Verification items for the finished model (mm, model axes). Face numbers are marked on the shaded views. A direction names the side the tool comes from. Coordinates: 2 decimals unless noted, no trailing zeros. Loops run counter-clockwise (first coordinate to the right, second up) from the corner with the lowest first, then second, coordinate; pieces in that order, holes last. Notation, with made-up numbers: (60.25, 1.5) - (105.25, 1.5) arc R15 ccw to (105.25, 8.5) - close; hole circle Ø6 at (-29, 11.5). An arc over 180 degrees is marked (long way). One line per item, written item: value. Start each with the question number.
(1) Section check C-C (x = 424.5). Record the boundary of the cut face in (y, z), plus the area to 3 significant figures.
(2) Gauge pin test, flat end, axial feed: P1, Ø8, axis at y = 115.5, z = 32, coming from the -X side. Record the tip position at first contact, or that the pin passes through.
(3) Draft check along Y on the marked faces 3, 4, 5 and 6. Enter one of: +Y half, -Y half, draft (parallel to the pull), parting line (faces both ways), or undercut.
(4) Section check A-A (z = 51). Record the boundary of the cut face in (x, y).
(5) Set-up check for the marked faces 1 and 2: record each of +Z, -Z, +X, -X, +Y, -Y from which the full face is reachable in a straight line by a thin tool's end or side.
(6) Thickness scan on probe 1 along Y at (x, z) = (173, 24); probe 2 along X at (y, z) = (34.5, 9); probe 3 along Y at (x, z) = (623, 72.5). Record the ranges inside material, lowest first. Write a range as [from, to].
(7) Section check B-B (y = -10.5). Record the boundary of the cut face in (x, z), plus the area to 3 significant figures.
Autodesk Inventor part; units mm, degrees
ref_plane "YZ Plane" through (0, 0, 0) normal (1, 0, 0) x (0, 1, 0)
ref_plane "XZ Plane" through (0, 0, 0) normal (0, 1, 0) x (-1, 0, 0)
ref_plane "XY Plane" through (0, 0, 0) normal (0, 0, 1) x (1, 0, 0)
sketch "Chassis" plane through (0, 0, 0) normal (0, 0, 1) x (1, 0, 0)
  line L0 (0, 0) -> (660.4, 0) construction
  line L1 (660.4, 0) -> (660.4, 152.4) construction
  line L2 (660.4, 152.4) -> (0, 152.4) construction
  line L3 (0, 152.4) -> (0, 0) construction
  line L4 (50.8, 127) -> (609.6, 127) construction
  line L5 (635, 101.6) -> (635, 50.8) construction
  line L6 (609.6, 25.4) -> (50.8, 25.4) construction
  line L7 (25.4, 50.8) -> (25.4, 101.6) construction
  arc A0 (50.8, 127) -> (25.4, 101.6) centre (50.8, 101.6) ccw construction
  arc A1 (25.4, 50.8) -> (50.8, 25.4) centre (50.8, 50.8) ccw construction
  arc A2 (609.6, 25.4) -> (635, 50.8) centre (609.6, 50.8) ccw construction
  arc A3 (635, 101.6) -> (609.6, 127) centre (609.6, 101.6) ccw construction
  dimension "d0" = 660.4
  dimension "d1" = 152.4
  dimension "d3" = 25.4
  dimension "d4" = 25.4
sketch "Motor and motor mount" plane through (0, 0, 0) normal (0, 0, 1) x (1, 0, 0)
  line L0 (152.5322, 25.4) -> (519.6657, 25.4) construction
  line L1 (519.6657, 25.4) -> (519.6657, 127) construction
  line L2 (519.6657, 127) -> (152.5322, 127) construction
  line L3 (152.5322, 127) -> (152.5322, 25.4) construction
  line L4 (152.5322, 31.75) -> (519.6657, 31.75) construction
  line L5 (168.5983, 31.75) -> (502.5549, 31.75) construction
  line L6 (502.5549, 31.75) -> (502.5549, 131.1076) construction
  line L7 (502.5549, 131.1076) -> (168.5983, 131.1076) construction
  line L8 (168.5983, 131.1076) -> (168.5983, 31.75) construction
  circle A0 centre (459.6569, 62.4006) radius 45.974 construction
  line L9 (50.8, 127) -> (609.6, 127) construction
  line L10 (168.5983, 121.0746) -> (502.5549, 121.0746) construction
  line L11 (76.2661, 152.2106) -> (76.2661, 127) construction
  line L12 (0, 152.4) -> (0, 0) construction
  line L13 (609.6, 25.4) -> (50.8, 25.4) construction
  circle A1 centre (459.6569, 62.4006) radius 6.35 construction
  point P0 (76.2661, 139.6053)
  dimension "d5" = 367.1334
  dimension "d6" = 101.6
  dimension "d8" = 6.35
  dimension "d9" = 333.9566
  dimension "d10" = 17.1108
  dimension "d12" = 42.898
  dimension "d14" = 4.1076
  dimension "d15" = 5.9254
  dimension "d16" = 58.674
  dimension "d17" = 76.2661
  dimension "d18" = 76.2661
  dimension "d19" = 91.948
  dimension "d20" = 12.7
sketch "Flipper drive rails" plane through (0, 0, 0) normal (0, 0, 1) x (1, 0, 0)
  circle A0 centre (609.6, 48.1766) radius 12.7 construction
  line L0 (660.4, 0) -> (660.4, 152.4) construction
  line L1 (0, 0) -> (660.4, 0) construction
  circle A1 centre (50.8, 48.1766) radius 12.7 construction
  line L2 (0, 152.4) -> (0, 0) construction
  circle A2 centre (50.8, 48.1766) radius 58.166 construction
  circle A3 centre (609.6, 48.1766) radius 58.166 construction
  circle A4 centre (459.6569, 62.4006) radius 45.974 construction
  dimension "d21" = 25.4
  dimension "d22" = 50.8
  dimension "d24" = 25.4
  dimension "d25" = 50.8
  dimension "d27" = 116.332
  dimension "d28" = 116.332
  dimension "d49" = 14.224
sketch "Flipper Gears" plane through (0, 0, 0) normal (0, 0, 1) x (1, 0, 0)
  circle A0 centre (172.9676, 98.1053) radius 29.845 construction
  circle A1 centre (217.0566, 68.0834) radius 23.495 construction
  circle A2 centre (132.7629, 49.7774) radius 33.02 construction
  circle A3 centre (132.7629, 49.7774) radius 23.8125 construction
  circle A4 centre (50.8, 48.1766) radius 58.166 construction
  circle A5 centre (609.6, 48.1766) radius 12.7 construction
  circle A6 centre (609.6, 48.1766) radius 86.36 construction
  circle A7 centre (502.1097, 24.0144) radius 23.8125 construction
  circle A8 centre (502.1097, 24.0144) radius 33.02 construction
  circle A9 centre (447.4639, 55.0924) radius 29.845 construction
  circle A10 centre (410.72, 16.4266) radius 23.495 construction
  line L0 (253.1246, 92.8334) -> (396.8286, 92.8334) construction
  line L1 (396.8286, 92.8334) -> (396.8286, 43.3334) construction
  line L2 (396.8286, 43.3334) -> (253.1246, 43.3334) construction
  line L3 (253.1246, 43.3334) -> (253.1246, 92.8334) construction
  line L4 (374.652, 16.4266) -> (410.72, 16.4266) construction
  line L5 (217.0566, 68.0834) -> (253.1246, 68.0834) construction
  line L6 (230.948, 41.1766) -> (374.652, 41.1766) construction
  line L7 (374.652, 41.1766) -> (374.652, -8.3234) construction
  line L8 (374.652, -8.3234) -> (230.948, -8.3234) construction
  line L9 (230.948, -8.3234) -> (230.948, 41.1766) construction
  circle A11 centre (50.8, 48.1766) radius 86.36 construction
  line L10 (50.8, 48.1766) -> (609.6, 48.1766) construction
  line L11 (50.8, -50.8834) -> (609.6, -50.8834) construction
  line L12 (609.6, 147.2366) -> (50.8, 147.2366) construction
  arc A12 (50.8, 147.2366) -> (50.8, -50.8834) centre (50.8, 48.1766) ccw construction
  arc A13 (609.6, -50.8834) -> (609.6, 147.2366) centre (609.6, 48.1766) ccw construction
  circle A14 centre (50.8, 48.1766) radius 99.06 construction
  line L13 (50.8, 48.1766) -> (609.6, 48.1766) construction
  line L14 (50.8, -38.1834) -> (609.6, -38.1834) construction
  line L15 (609.6, 134.5366) -> (50.8, 134.5366) construction
  arc A15 (50.8, 134.5366) -> (50.8, -38.1834) centre (50.8, 48.1766) ccw construction
  arc A16 (609.6, -38.1834) -> (609.6, 134.5366) centre (609.6, 48.1766) ccw construction
  point P0 (0, 0)
  point P1 (330.2, 48.1766)
  point P2 (330.2, 48.1766)
  dimension "d29" = 59.69
  dimension "d30" = 46.99
  dimension "d31" = 66.04
  dimension "d32" = 47.625
  dimension "d34" = 172.72
  dimension "d35" = 47.625
  dimension "d36" = 66.04
  dimension "d37" = 59.69
  dimension "d38" = 46.99
  dimension "d39" = 143.704
  dimension "d40" = 49.5
  dimension "d43" = 36.068
  dimension "d48" = 24.1623
  dimension "d50" = 31.75
  dimension "d51" = 38.6658
  dimension "d52" = 143.704
  dimension "d53" = 49.5
  dimension "d54" = 36.068
  dimension "d55" = 51.6568
  dimension "d60" = 172.72
  dimension "d62" = 12.7
sketch "Flipper" plane through (0, 0, 0) normal (0, 0, 1) x (1, 0, 0)
  circle A0 centre (50.8, 48.1766) radius 63.5 construction
  circle A1 centre (-195.1482, 3.0916) radius 41.275 construction
  circle A2 centre (50.8, 48.1766) radius 86.36 construction
  line L0 (-195.1482, -38.1834) -> (50.8, -38.1834) construction
  point P0 (0, 0)
  point P1 (609.6, 48.1766)
  dimension "d57" = 82.55
  dimension "d58" = 172.72
  dimension "d56" = 127
  dimension "d59" = 245.9482
sketch "Sketch6" plane through (0, 0, 0) normal (0, 0, 1) x (1, 0, 0)
  line L0 (609.6, 147.2366) -> (50.8, 147.2366)
  arc A0 (50.8, 147.2366) -> (50.8, -50.8834) centre (50.8, 48.1766) ccw
  line L1 (609.6, 134.5366) -> (50.8, 134.5366)
  circle A1 centre (50.8, 48.1766) radius 86.36
  line L2 (50.8, -38.1834) -> (609.6, -38.1834)
  line L3 (50.8, -50.8834) -> (609.6, -50.8834)
  arc A2 (609.6, -50.8834) -> (609.6, 147.2366) centre (609.6, 48.1766) ccw
  circle A3 centre (609.6, 48.1766) radius 86.36
  point P0 (0, 0)
extrude "Extrusion1" add sketch "Sketch6" along normal blind 76.2
properties part number "MasterSketch"
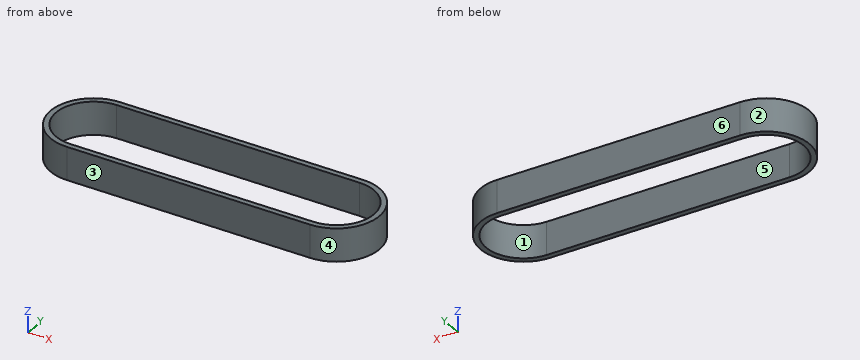
Responses:
1. outline: (-50.88, 0) - (-38.18, 0) - (-38.18, 76.2) - (-50.88, 76.2) - close; (134.54, 0) - (147.24, 0) - (147.24, 76.2) - (134.54, 76.2) - close
1. area: 1,940 mm²
2. P1: stops at x = -25.38
3. face 3: -Y half
3. face 4: parting line
3. face 5: undercut
3. face 6: +Y half
4. outline: (50.8, -50.88) - (609.6, -50.88) arc R99.06 ccw to (609.6, 147.24) - (50.8, 147.24) arc R99.06 ccw to start; hole (50.8, -38.18) - (609.6, -38.18) arc R86.36 ccw to (609.6, 134.54) - (50.8, 134.54) arc R86.36 ccw to start
5. face 1: +Z, -Z
5. face 2: +Z, -Z, -X
6. probe 1: y = [-50.88, -38.18], [134.54, 147.24]
6. probe 2: x = [-47.31, -34.47], [694.87, 707.71]
6. probe 3: y = [-49.97, -37.14], [133.49, 146.33]
7. outline: (-29.01, 0) - (-12.56, 0) - (-12.56, 76.2) - (-29.01, 76.2) - close; (672.96, 0) - (689.41, 0) - (689.41, 76.2) - (672.96, 76.2) - close
7. area: 2,510 mm²
